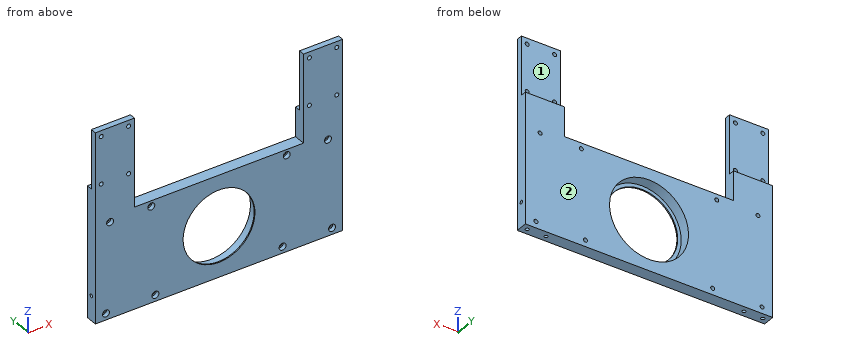
```python
from build123d import *

# Parameters (mm, degrees)
SKIZZE1_W                        = 210
SKIZZE1_H                        = 400
AUFSATZ_LINEAR_AUSTRAGEN1_DEPTH  = 10
SKIZZE5_W                        = 210
SKIZZE5_H                        = 85
SCHNITT_LINEAR_AUSTRAGEN2_DEPTH  = 10
SKIZZE6_R                        = 1.7
SCHNITT_LINEAR_AUSTRAGEN3_DEPTH  = 227.108381092
SCHNITT_LINEAR_AUSTRAGEN4_DEPTH  = 4
SKIZZE16_W                       = 35
SKIZZE16_H                       = 7
SCHNITT_LINEAR_AUSTRAGEN10_DEPTH = 5
SCHNITT_LINEAR_AUSTRAGEN11_DEPTH = 35
SKIZZE20_R                       = 1.7
SCHNITT_LINEAR_AUSTRAGEN12_DEPTH = 227.108381092
SKIZZE21_W                       = 143.493506494
SKIZZE21_H                       = 75
SCHNITT_LINEAR_AUSTRAGEN13_DEPTH = 227.108381092
SCHNITT_LINEAR_AUSTRAGEN14_DEPTH = 227.108381092
AUFSATZ_LINEAR_AUSTRAGEN6_DEPTH  = 10
SKIZZE25_R                       = 1.7
SCHNITT_LINEAR_AUSTRAGEN15_DEPTH = 227.108381092
SCHNITT_LINEAR_AUSTRAGEN16_DEPTH = 291.172362571
SKIZZE27_R                       = 33.5
SCHNITT_LINEAR_AUSTRAGEN17_DEPTH = 157.044865343
SKIZZE28_R                       = 36.006256149
SKIZZE28_R_2                     = 30.5
AUFSATZ_LINEAR_AUSTRAGEN7_DEPTH  = 1
SKIZZE29_R                       = 1.5
SCHNITT_LINEAR_AUSTRAGEN18_DEPTH = 10
SKIZZE30_R                       = 1.5
SCHNITT_LINEAR_AUSTRAGEN19_DEPTH = 10
SKIZZE31_R                       = 2.95
SCHNITT_LINEAR_AUSTRAGEN20_DEPTH = 3.5


with BuildPart() as part:
    # Skizze1 → Aufsatz-Linear austragen1 (new body)
    with BuildSketch(Plane(origin=(0, 0, 0), x_dir=(1, 0, 0), z_dir=(0, 1, 0))):
        Rectangle(SKIZZE1_W, SKIZZE1_H)
    extrude(amount=AUFSATZ_LINEAR_AUSTRAGEN1_DEPTH)

    # Skizze5 → Schnitt-Linear austragen2 (cut)
    with BuildSketch(Plane(origin=(0, 10, 0), x_dir=(1, 0, 0), z_dir=(0, 1, 0))):
        Polygon((105, -200), (18, -200), (105, -46), align=None)
        Polygon((-18, -200), (-105, -46), (-105, -200), align=None)
        with Locations((0, 157.5)):
            Rectangle(SKIZZE5_W, SKIZZE5_H)
        Polygon((71.746753247, -46), (-71.746753247, -46), (-2.824675325, -168), (2.824675325, -168), align=None)
    extrude(amount=-SCHNITT_LINEAR_AUSTRAGEN2_DEPTH, mode=Mode.SUBTRACT)

    # Skizze6 → Schnitt-Linear austragen3 (cut, through all)
    with BuildSketch(Plane(origin=(0, 10, 0), x_dir=(1, 0, 0), z_dir=(0, 1, 0))):
        with Locations(Location((-11, -195, 0), (0, 0, 270))):
            Circle(SKIZZE6_R)
        with Locations(Location((-11, -178.18, 0), (0, 0, 90))):
            Circle(SKIZZE6_R)
        with Locations(Location((11, -195, 0), (0, 0, 90))):
            Circle(SKIZZE6_R)
        with Locations(Location((11, -178.18, 0), (0, 0, 270))):
            Circle(SKIZZE6_R)
    extrude(amount=-SCHNITT_LINEAR_AUSTRAGEN3_DEPTH, mode=Mode.SUBTRACT)

    # Skizze7 → Schnitt-Linear austragen4 (cut)
    with BuildSketch(Plane.XZ):
        Polygon((-11, 198.406366588), (-8.05, 196.703183294), (-8.05, 193.296816706), (-11, 191.593633412), (-13.95, 193.296816706), (-13.95, 196.703183294), align=None)
        Polygon((11, 198.406366588), (8.05, 196.703183294), (8.05, 193.296816706), (11, 191.593633412), (13.95, 193.296816706), (13.95, 196.703183294), align=None)
        Polygon((-8.05, 176.476816706), (-8.05, 179.883183294), (-11, 181.586366588), (-13.95, 179.883183294), (-13.95, 176.476816706), (-11, 174.773633412), align=None)
        Polygon((8.05, 176.476816706), (8.05, 179.883183294), (11, 181.586366588), (13.95, 179.883183294), (13.95, 176.476816706), (11, 174.773633412), align=None)
    extrude(amount=-SCHNITT_LINEAR_AUSTRAGEN4_DEPTH, mode=Mode.SUBTRACT)

    # Skizze16 → Schnitt-Linear austragen10 (cut)
    with BuildSketch(Plane.XZ):
        with Locations((0, 186.59)):
            Rectangle(SKIZZE16_W, SKIZZE16_H)
    extrude(amount=-SCHNITT_LINEAR_AUSTRAGEN10_DEPTH, mode=Mode.SUBTRACT)

    # Skizze17 → Schnitt-Linear austragen11 (cut)
    with BuildSketch(Plane.ZY.offset(-17.5)):
        Polygon((183.09, 5), (186.59, 8.5), (190.09, 5), align=None)
    extrude(amount=SCHNITT_LINEAR_AUSTRAGEN11_DEPTH, mode=Mode.SUBTRACT)

    # Skizze20 → Schnitt-Linear austragen12 (cut, through all)
    with BuildSketch(Plane(origin=(0, 10, 0), x_dir=(1, 0, 0), z_dir=(0, 1, 0))):
        with Locations(Location((96, 109.52, 0), (0, 0, 270))):
            Circle(SKIZZE20_R)
        with Locations(Location((54, 109.52, 0), (0, 0, 270))):
            Circle(SKIZZE20_R)
        with Locations(Location((-54, 109.52, 0), (0, 0, 90))):
            Circle(SKIZZE20_R)
        with Locations(Location((-96, 109.52, 0), (0, 0, 90))):
            Circle(SKIZZE20_R)
        with Locations(Location((92.5, 33.82, 0), (0, 0, 270))):
            Circle(SKIZZE20_R)
        with Locations(Location((57.5, 33.82, 0), (0, 0, 270))):
            Circle(SKIZZE20_R)
        with Locations(Location((-92.5, 33.82, 0), (0, 0, 90))):
            Circle(SKIZZE20_R)
        with Locations(Location((-57.5, 33.82, 0), (0, 0, 90))):
            Circle(SKIZZE20_R)
    extrude(amount=-SCHNITT_LINEAR_AUSTRAGEN12_DEPTH, mode=Mode.SUBTRACT)

    # Skizze21 → Schnitt-Linear austragen13 (cut, through all)
    with BuildSketch(Plane(origin=(0, 10, 0), x_dir=(1, 0, 0), z_dir=(0, 1, 0))):
        with Locations((0, -8.5)):
            Rectangle(SKIZZE21_W, SKIZZE21_H)
    extrude(amount=-SCHNITT_LINEAR_AUSTRAGEN13_DEPTH, mode=Mode.SUBTRACT)

    # Skizze22 → Schnitt-Linear austragen14 (cut, through all)
    with BuildSketch(Plane(origin=(0, 10, 0), x_dir=(1, 0, 0), z_dir=(0, 1, 0))):
        with BuildLine():
            Line((-71.746753247, -46), (-2.824675325, -168))
            ThreePointArc((-2.824675325, -168), (-55.506711033, -117.293679981), (-71.746753247, -46))
        make_face()
    schnitt_linear_austragen14 = extrude(amount=-SCHNITT_LINEAR_AUSTRAGEN14_DEPTH, mode=Mode.SUBTRACT)

    # Skizze23 → Aufsatz-Linear austragen6 (add)
    with BuildSketch(Plane(origin=(0, 10, 0), x_dir=(1, 0, 0), z_dir=(0, 1, 0))):
        with BuildLine():
            Line((-105, -46), (-18, -200))
            ThreePointArc((-18, -200), (-78.088357737, -132.371344955), (-105, -46))
        make_face()
    aufsatz_linear_austragen6 = extrude(amount=-AUFSATZ_LINEAR_AUSTRAGEN6_DEPTH)

    # Spiegeln2: Schnitt-Linear austragen14, Aufsatz-Linear austragen6 across plane
    add(schnitt_linear_austragen14.mirror(Plane(origin=(0, 0, 0), x_dir=(0, 0, 1), z_dir=(1, 0, 0))), mode=Mode.SUBTRACT)
    add(aufsatz_linear_austragen6.mirror(Plane(origin=(0, 0, 0), x_dir=(0, 0, 1), z_dir=(1, 0, 0))))

    # Skizze25 → Schnitt-Linear austragen15 (cut, through all)
    with BuildSketch(Plane(origin=(0, 10, 0), x_dir=(1, 0, 0), z_dir=(0, 1, 0))):
        with Locations(Location((-100, -1, 0), (0, 0, 270))):
            Circle(SKIZZE25_R)
        with Locations(Location((-76.746753247, -1, 0), (0, 0, 90))):
            Circle(SKIZZE25_R)
        with Locations(Location((-76.746753247, -41, 0), (0, 0, 270))):
            Circle(SKIZZE25_R)
        with Locations(Location((-100, -41, 0), (0, 0, 90))):
            Circle(SKIZZE25_R)
    schnitt_linear_austragen15 = extrude(amount=-SCHNITT_LINEAR_AUSTRAGEN15_DEPTH, mode=Mode.SUBTRACT)

    # Spiegeln3: Schnitt-Linear austragen15 across plane
    add(schnitt_linear_austragen15.mirror(Plane(origin=(0, 0, 0), x_dir=(0, 0, 1), z_dir=(1, 0, 0))), mode=Mode.SUBTRACT)

    # Skizze26 → Schnitt-Linear austragen16 (cut, through all)
    with BuildSketch(Plane.ZY.offset(105)):
        Polygon((-4, 5), (-4, 13.101486595), (200.684563047, 82.546277137), (242.997216492, -41.037631402), (91.241487897, -60.284782055), (46, 0), (46, 5), align=None)
    extrude(amount=-SCHNITT_LINEAR_AUSTRAGEN16_DEPTH, mode=Mode.SUBTRACT)

    # Skizze27 → Schnitt-Linear austragen17 (cut, through all)
    with BuildSketch(Plane(origin=(0, 10, 0), x_dir=(1, 0, 0), z_dir=(0, 1, 0))):
        with Locations(Location((0, 72, 0), (0, 0, 270))):
            Circle(SKIZZE27_R)
    extrude(amount=-SCHNITT_LINEAR_AUSTRAGEN17_DEPTH, mode=Mode.SUBTRACT)

    # Skizze28 → Aufsatz-Linear austragen7 (add)
    with BuildSketch(Plane.XZ):
        with Locations((0, -72)):
            Circle(SKIZZE28_R)
        with Locations(Location((0, -72, 0), (0, 0, 270))):
            Circle(SKIZZE28_R_2, mode=Mode.SUBTRACT)
    extrude(amount=-AUFSATZ_LINEAR_AUSTRAGEN7_DEPTH)

    # Skizze29 → Schnitt-Linear austragen18 (cut)
    with BuildSketch(Plane.ZY.offset(105)):
        with Locations((-94, 5)):
            Circle(SKIZZE29_R)
    schnitt_linear_austragen18 = extrude(amount=-SCHNITT_LINEAR_AUSTRAGEN18_DEPTH, mode=Mode.SUBTRACT)

    # Skizze30 → Schnitt-Linear austragen19 (cut)
    with BuildSketch(Plane(origin=(0, 0, -115), x_dir=(-1, 0, 0), z_dir=(0, 0, -1))):
        with Locations((100, 5)):
            Circle(SKIZZE30_R)
        with Locations((84, 5)):
            Circle(SKIZZE30_R)
    schnitt_linear_austragen19 = extrude(amount=-SCHNITT_LINEAR_AUSTRAGEN19_DEPTH, mode=Mode.SUBTRACT)

    # Spiegeln4: Schnitt-Linear austragen18, Schnitt-Linear austragen19 across plane
    add(schnitt_linear_austragen18.mirror(Plane(origin=(0, 0, 0), x_dir=(0, 0, 1), z_dir=(1, 0, 0))), mode=Mode.SUBTRACT)
    add(schnitt_linear_austragen19.mirror(Plane(origin=(0, 0, 0), x_dir=(0, 0, 1), z_dir=(1, 0, 0))), mode=Mode.SUBTRACT)

    # Skizze31 → Schnitt-Linear austragen20 (cut)
    with BuildSketch(Plane.XZ):
        with Locations(Location((-96, -109.52, 0), (0, 0, 270))):
            Circle(SKIZZE31_R)
        with Locations(Location((-54, -109.52, 0), (0, 0, 270))):
            Circle(SKIZZE31_R)
        with Locations(Location((-92.5, -33.82, 0), (0, 0, 270))):
            Circle(SKIZZE31_R)
        with Locations(Location((-57.5, -33.82, 0), (0, 0, 270))):
            Circle(SKIZZE31_R)
        with Locations(Location((57.5, -33.82, 0), (0, 0, 90))):
            Circle(SKIZZE31_R)
        with Locations(Location((92.5, -33.82, 0), (0, 0, 90))):
            Circle(SKIZZE31_R)
        with Locations(Location((54, -109.52, 0), (0, 0, 90))):
            Circle(SKIZZE31_R)
        with Locations(Location((96, -109.52, 0), (0, 0, 90))):
            Circle(SKIZZE31_R)
    extrude(amount=-SCHNITT_LINEAR_AUSTRAGEN20_DEPTH, mode=Mode.SUBTRACT)


solid = part.part
```
For this review, take the finished solid that the model builds, in its own axes (mm). Face numbers are marked on the shaded views. A direction names the side the tool comes from. Round coordinates to 2 decimals unless told otherwise and drop trailing zeros. Order: outer loops, then holes, each group sorted by start corner. A loop starts at its lowest first (then second) coordinate and runs counter-clockwise, first axis right, second up.
Q1. Insertion check: P1, Ø4, axis at x = 89, y = 7.5, coming from the +Z side; P2, Ø1.8, axis at x = 92.5, z = -35, coming from the -Y side; P3, Ø5.5, axis at x = -100, z = 41, coming from the +Y side. Each pin has a flat end and moves straight along its axis. Give the tip position at first contact, or say it passes through.
Findings below:
P1: stops at z = -4
P2: stops at y = 3.5
P3: stops at y = 5
Q2. Wall thickness on line 1 (Z direction, x = 100, y = 2.4); line 2 (X direction, y = 8.5, z = -109.52); line 3 (Z direction, x = -92.5, y = 7.75): over which ranges is each line inside the solid? List them lowest first.
Findings below:
line 1: z = -115 to -0.7, 2.7 to 39.3, 42.7 to 46
line 2: x = -105 to -97.7, -94.3 to -55.7, -52.3 to 52.3, 55.7 to 94.3, 97.7 to 105
line 3: z = -115 to -35.52, -32.12 to -4
Q3. Machinability: for the marked faces 1 and 2, which of the approach directions +Z, -Z, +X, -X, +Y, -Y give a long, thin tool a straight path to every point of the face, cutting with its end or side? Answer none if there is none.
Findings below:
face 1: +Z, +X, -X, +Y
face 2: +Z, -Z, +X, -X, +Y
Q4. We need section A-A, the plane z = -72. Give the boundary of the cut face in (x, y).
Findings below:
outline: (-105, 0) - (-30.5, 0) - (-30.5, 1) - (-33.5, 1) - (-33.5, 10) - (-105, 10) - close; (30.5, 0) - (105, 0) - (105, 10) - (33.5, 10) - (33.5, 1) - (30.5, 1) - close
Q5. We need section C-C, the plane z = -26. Give the boundary of the cut face in (x, y).
Findings below:
outline: (-105, 0) - (-71.75, 0) - (-71.75, 10) - (-105, 10) - close; (71.75, 0) - (105, 0) - (105, 10) - (71.75, 10) - close
Q6. We need section D-D, the plane z = 7. Give the boundary of the cut face in (x, y), plus the area to 3 significant figures.
Findings below:
outline: (-105, 0) - (-71.75, 0) - (-71.75, 5) - (-105, 5) - close; (71.75, 0) - (105, 0) - (105, 5) - (71.75, 5) - close
area: 333 mm2
Q7. We need section B-B, the plane x = -26. Give the boundary of the cut face in (y, z), plus the area to 3 significant figures.
Findings below:
outline: (0, -115) - (10, -115) - (10, -93.12) - (1, -93.12) - (1, -87.95) - (0, -87.95) - close; (0, -56.05) - (1, -56.05) - (1, -50.88) - (10, -50.88) - (10, -29) - (0, -29) - close
area: 448 mm2
